```python
from build123d import *

# Parameters (mm, degrees)
SKETCH2_R           = 50
SKETCH2_R_2         = 6.5
BOSS_EXTRUDE1_DEPTH = 25
CUT_EXTRUDE1_DEPTH  = 76


with BuildPart() as part:
    # Sketch2 → Boss-Extrude1 (new body)
    with BuildSketch(Plane(origin=(0, 0, 0), x_dir=(0, 1, 0), z_dir=(0, 0, 1))):
        with Locations(Location((0, 0, 0), (0, 0, 270))):
            Circle(SKETCH2_R)
        with Locations(Location((0, 42, 0), (0, 0, 270))):
            Circle(SKETCH2_R_2, mode=Mode.SUBTRACT)
        with Locations(Location((29.69848481, 29.69848481, 0), (0, 0, 270))):
            Circle(SKETCH2_R_2, mode=Mode.SUBTRACT)
        with Locations(Location((42, 0, 0), (0, 0, 270))):
            Circle(SKETCH2_R_2, mode=Mode.SUBTRACT)
        with Locations(Location((29.69848481, -29.69848481, 0), (0, 0, 270))):
            Circle(SKETCH2_R_2, mode=Mode.SUBTRACT)
        with Locations(Location((0, -42, 0), (0, 0, 270))):
            Circle(SKETCH2_R_2, mode=Mode.SUBTRACT)
        with Locations(Location((-29.69848481, -29.69848481, 0), (0, 0, 270))):
            Circle(SKETCH2_R_2, mode=Mode.SUBTRACT)
        with Locations(Location((-42, 0, 0), (0, 0, 270))):
            Circle(SKETCH2_R_2, mode=Mode.SUBTRACT)
        with Locations(Location((-29.69848481, 29.69848481, 0), (0, 0, 270))):
            Circle(SKETCH2_R_2, mode=Mode.SUBTRACT)
        with Locations(Location((-38.802940365, 16.072704159, 0), (0, 0, 270))):
            Circle(SKETCH2_R_2, mode=Mode.SUBTRACT)
        with Locations(Location((-16.072704159, 38.802940365, 0), (0, 0, 270))):
            Circle(SKETCH2_R_2, mode=Mode.SUBTRACT)
        with Locations(Location((16.072704159, 38.802940365, 0), (0, 0, 270))):
            Circle(SKETCH2_R_2, mode=Mode.SUBTRACT)
        with Locations(Location((38.802940365, 16.072704159, 0), (0, 0, 270))):
            Circle(SKETCH2_R_2, mode=Mode.SUBTRACT)
        with Locations(Location((38.802940365, -16.072704159, 0), (0, 0, 270))):
            Circle(SKETCH2_R_2, mode=Mode.SUBTRACT)
        with Locations(Location((16.072704159, -38.802940365, 0), (0, 0, 270))):
            Circle(SKETCH2_R_2, mode=Mode.SUBTRACT)
        with Locations(Location((-16.072704159, -38.802940365, 0), (0, 0, 270))):
            Circle(SKETCH2_R_2, mode=Mode.SUBTRACT)
        with Locations(Location((-38.802940365, -16.072704159, 0), (0, 0, 270))):
            Circle(SKETCH2_R_2, mode=Mode.SUBTRACT)
    extrude(amount=BOSS_EXTRUDE1_DEPTH)

    # Sketch4 → Cut-Extrude1 (cut, through all)
    with BuildSketch(Plane.XY.offset(25)):
        with BuildLine():
            Line((-0.5, 4), (0.5, 4))
            Line((0.5, 4), (0.5, 2.958039892))
            ThreePointArc((0.5, 2.958039892), (0.776457135, 2.897777479), (1.046007244, 2.811737691))
            Line((1.046007244, 2.811737691), (1.566987298, 3.714101615))
            Line((1.566987298, 3.714101615), (2.433012702, 3.214101615))
            Line((2.433012702, 3.214101615), (1.912032648, 2.311737691))
            ThreePointArc((1.912032648, 2.311737691), (2.121320344, 2.121320344), (2.311737691, 1.912032648))
            Line((2.311737691, 1.912032648), (3.214101615, 2.433012702))
            Line((3.214101615, 2.433012702), (3.714101615, 1.566987298))
            Line((3.714101615, 1.566987298), (2.811737691, 1.046007244))
            ThreePointArc((2.811737691, 1.046007244), (2.897777479, 0.776457135), (2.958039892, 0.5))
            Line((2.958039892, 0.5), (4, 0.5))
            Line((4, 0.5), (4, -0.5))
            Line((4, -0.5), (2.958039892, -0.5))
            ThreePointArc((2.958039892, -0.5), (2.897777479, -0.776457135), (2.811737691, -1.046007244))
            Line((2.811737691, -1.046007244), (3.714101615, -1.566987298))
            Line((3.714101615, -1.566987298), (3.214101615, -2.433012702))
            Line((3.214101615, -2.433012702), (2.311737691, -1.912032648))
            ThreePointArc((2.311737691, -1.912032648), (2.121320344, -2.121320344), (1.912032648, -2.311737691))
            Line((1.912032648, -2.311737691), (2.433012702, -3.214101615))
            Line((2.433012702, -3.214101615), (1.566987298, -3.714101615))
            Line((1.566987298, -3.714101615), (1.046007244, -2.811737691))
            ThreePointArc((1.046007244, -2.811737691), (0.776457135, -2.897777479), (0.5, -2.958039892))
            Line((0.5, -2.958039892), (0.5, -4))
            Line((0.5, -4), (-0.5, -4))
            Line((-0.5, -4), (-0.5, -2.958039892))
            ThreePointArc((-0.5, -2.958039892), (-0.776457135, -2.897777479), (-1.046007244, -2.811737691))
            Line((-1.046007244, -2.811737691), (-1.566987298, -3.714101615))
            Line((-1.566987298, -3.714101615), (-2.433012702, -3.214101615))
            Line((-2.433012702, -3.214101615), (-1.912032648, -2.311737691))
            ThreePointArc((-1.912032648, -2.311737691), (-2.121320344, -2.121320344), (-2.311737691, -1.912032648))
            Line((-2.311737691, -1.912032648), (-3.214101615, -2.433012702))
            Line((-3.214101615, -2.433012702), (-3.714101615, -1.566987298))
            Line((-3.714101615, -1.566987298), (-2.811737691, -1.046007244))
            ThreePointArc((-2.811737691, -1.046007244), (-2.897777479, -0.776457135), (-2.958039892, -0.5))
            Line((-2.958039892, -0.5), (-4, -0.5))
            Line((-4, -0.5), (-4, 0.5))
            Line((-4, 0.5), (-2.958039892, 0.5))
            ThreePointArc((-2.958039892, 0.5), (-2.897777479, 0.776457135), (-2.811737691, 1.046007244))
            Line((-2.811737691, 1.046007244), (-3.714101615, 1.566987298))
            Line((-3.714101615, 1.566987298), (-3.214101615, 2.433012702))
            Line((-3.214101615, 2.433012702), (-2.311737691, 1.912032648))
            ThreePointArc((-2.311737691, 1.912032648), (-2.121320344, 2.121320344), (-1.912032648, 2.311737691))
            Line((-1.912032648, 2.311737691), (-2.433012702, 3.214101615))
            Line((-2.433012702, 3.214101615), (-1.566987298, 3.714101615))
            Line((-1.566987298, 3.714101615), (-1.046007244, 2.811737691))
            ThreePointArc((-1.046007244, 2.811737691), (-0.776457135, 2.897777479), (-0.5, 2.958039892))
            Line((-0.5, 2.958039892), (-0.5, 4))
        make_face()
    extrude(amount=-CUT_EXTRUDE1_DEPTH, mode=Mode.SUBTRACT)


solid = part.part
```
CAD build for the part. Positions are in the model's coordinates, mm. Coordinates: 2 decimals unless noted, no trailing zeros. Write each loop counter-clockwise with the first axis right and the second up, starting at its lowest first coordinate (ties: lowest second). Pieces come first, ordered by that corner, then holes. Notation, with made-up numbers: (15.5, -38.75) -> (47.5, -38.75) arc R14 cw to (47.5, -21.75) -> close; hole circle Ø9 at (89.5, -27). An arc over 180 degrees is marked (long way). Use CSV: the item, a comma, the result in double quotes. Start each with the question number.
Item 1: Drop flat-ended pins along their axis: P1, Ø2, axis at y = -5, z = 22.5, coming from the -X side; P2, Ø4, axis at x = -30.5, z = 4.5, coming from the +Y side; P3, Ø1.5, axis at x = 12, z = 6, coming from the -Y side; P4, Ø8, axis at x = -38.8, y = -16.07, coming from the +Z side. Give the stop position or say it passes through.
Item 2: Band-saw the part on C-C, the plane x = 42.5. Write the cut outline in (y, z).
Item 3: Band-saw the part on B-B, the plane y = -11.5. Write the cut outline in (x, z), plus the area to 3 significant figures.
Item 4: Two-plate mould, pull along X, no slides. Class faces 1 (the flat face through (-1, -10, 0)), 2 (the cylindrical face through (-32.603, -14.12, 12.325)), 3 (the cylindrical face through (47.69, 15.02, 12.32)): +X half, -X half, draft (parallel to the pull), parting line (faces both ways), or undercut.
Item 5: Band-saw the part on D-D, the plane y = 42. Write the cut outline in (x, z), plus the area to 3 significant figures.
Item 6: Wall check: probe 1 along X at (y, z) = (-14, 14); probe 2 along X at (y, z) = (-44, 8.25); probe 3 along X at (y, z) = (18, 19.75). Give the ranges that are in metal, low to high.
Item 7: Band-saw the part on A-A, the plane x = 29.5. Write the cut outline in (y, z).
Response values:
1,P1,"stops at x = -49.84"
1,P2,"stops at y = 41.08"
1,P3,"stops at y = -48.72"
1,P4,"passes through"
2,outline,"(-26.34, 0) -> (-21.42, 0) -> (-21.42, 25) -> (-26.34, 25) -> close; (-10.73, 0) -> (-6.48, 0) -> (-6.48, 25) -> (-10.73, 25) -> close; (6.48, 0) -> (10.73, 0) -> (10.73, 25) -> (6.48, 25) -> close; (21.42, 0) -> (26.34, 0) -> (26.34, 25) -> (21.42, 25) -> close"
3,outline,"(-48.66, 0) -> (-43.42, 0) -> (-43.42, 25) -> (-48.66, 25) -> close; (-34.18, 0) -> (34.18, 0) -> (34.18, 25) -> (-34.18, 25) -> close; (43.42, 0) -> (48.66, 0) -> (48.66, 25) -> (43.42, 25) -> close"
3,area,"1,970 mm2"
4,face 1,"draft"
4,face 2,"undercut"
4,face 3,"parting line"
5,outline,"(-27.13, 0) -> (-21.73, 0) -> (-21.73, 25) -> (-27.13, 25) -> close; (-10.41, 0) -> (-6.5, 0) -> (-6.5, 25) -> (-10.41, 25) -> close; (6.5, 0) -> (10.41, 0) -> (10.41, 25) -> (6.5, 25) -> close; (21.73, 0) -> (27.13, 0) -> (27.13, 25) -> (21.73, 25) -> close"
5,area,"466 mm2"
6,probe 1,"x = -48 to -44.96, -32.64 to 32.64, 44.96 to 48"
6,probe 2,"x = -23.75 to -19.98, -12.17 to -6.18, 6.18 to 12.17, 19.98 to 23.75"
6,probe 3,"x = -46.65 to -45.01, -32.6 to 32.6, 45.01 to 46.65"
7,outline,"(-40.37, 0) -> (-36.2, 0) -> (-36.2, 25) -> (-40.37, 25) -> close; (-23.2, 0) -> (23.2, 0) -> (23.2, 25) -> (-23.2, 25) -> close; (36.2, 0) -> (40.37, 0) -> (40.37, 25) -> (36.2, 25) -> close"
